Autodesk Inventor part; units mm, degrees
ref_plane "YZ Plane" through (0, 0, 0) normal (1, 0, 0) x (0, 1, 0)
ref_plane "XZ Plane" through (0, 0, 0) normal (0, 1, 0) x (-1, 0, 0)
ref_plane "XY Plane" through (0, 0, 0) normal (0, 0, 1) x (1, 0, 0)
sketch "Sketch1" plane through (0, 0, 0) normal (0, 0, 1) x (1, 0, 0)
  line L0 (0, 0) -> (40, 0)
  line L1 (40, 0) -> (40, 10)
  line L2 (40, 10) -> (0, 10)
  line L3 (0, 10) -> (0, 0)
  dimension "d0" = 40
  dimension "d1" = 10
extrude "Extrusion1" add sketch "Sketch1" along normal blind 10
sketch "Sketch2" plane through (0, 0, 10) normal (0, 0, 1) x (1, 0, 0)
  line L0 (0, 10) -> (0, 0)
  line L1 (40, 10) -> (0, 10)
  point P0 (5, 5)
  point P1 (35, 5)
  dimension "d4" = 30
  dimension "d5" = 5
  dimension "d6" = 5
  dimension "d7" = 5
hole "Hole1" at (5, 5, 10) at (35, 5, 10) direction (0, 0, -1) diameter 6 depth 5 tip angle 118
sketch "Sketch3" plane through (0, 0, 0) normal (0, 0, -1) x (-1, 0, 0)
  line L0 (0, 0) -> (-40, 0)
  line L1 (0, 10) -> (0, 0)
  line L2 (-40, 10) -> (0, 10)
  line L3 (-40, 0) -> (-40, 10)
extrude "Extrusion2" add sketch "Sketch3" along normal blind 10
sketch "Sketch4" plane through (0, 0, 10) normal (0, -1, 0) x (1, 0, 0)
  line L0 (40, -20) -> (0, -20)
  line L1 (0, -20) -> (0, -23)
  line L2 (0, -23) -> (40, -23)
  line L3 (40, -23) -> (40, -20)
  point P0 (0, -10)
  dimension "d17" = 3
extrude "Extrusion3" add sketch "Sketch4" against normal blind 52
sketch "Sketch5" plane through (40, 0, -13) normal (0, 0, -1) x (-1, 0, 0)
  line L0 (0, 52) -> (40, 52)
  line L1 (40, 52) -> (40, 62)
  line L2 (40, 62) -> (0, 62)
  line L3 (0, 62) -> (0, 52)
  point P0 (40, 0)
  dimension "d20" = 10
extrude "Extrusion4" add sketch "Sketch5" against normal up to surface (23 mm away)
sketch "Sketch6" plane through (0, 10, 10) normal (0, 1, 0) x (1, 0, 0)
  line L0 (0, 20) -> (0, 0)
  line L1 (40, 0) -> (0, 0)
  line L2 (40, 20) -> (40, 0)
  line L3 (0, 20) -> (40, 20)
  point P0 (0, 10)
extrude "Extrusion5" add sketch "Sketch6" along normal blind 22
sketch "Sketch7" plane through (0, 0, 10) normal (0, 0, 1) x (1, 0, 0)
  circle A0 centre (5, 5) radius 3
  circle A1 centre (35, 5) radius 3
  line L0 (0, 0) -> (40, 0)
  line L1 (40, 0) -> (40, 32)
  line L2 (0, 32) -> (40, 32)
  line L3 (0, 0) -> (0, 32)
  line L4 (0, 52) -> (0, 62)
  line L5 (40, 52) -> (0, 52)
  line L6 (40, 62) -> (40, 52)
  line L7 (0, 62) -> (40, 62)
extrude "Extrusion6" add sketch "Sketch7" along normal blind 10
properties part number "rail mount"
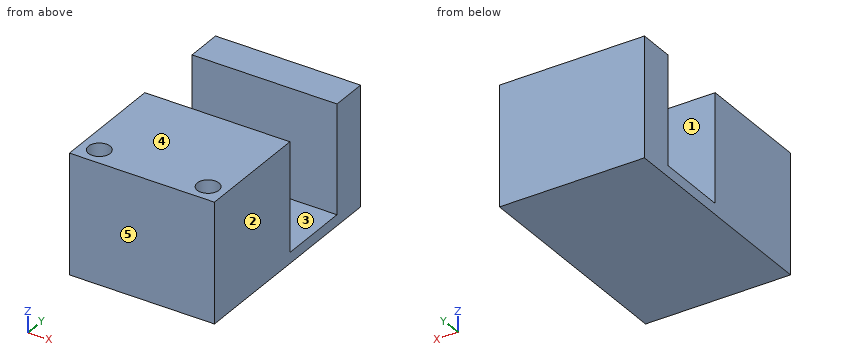
Design review of the part built by this model. Coordinates are the model's own, in mm. Face numbers are marked on the shaded views. A direction names the side the tool comes from. Round coordinates to 2 decimals unless told otherwise and drop trailing zeros. Write each loop counter-clockwise with the first axis right and the second up, starting at its lowest first coordinate (ties: lowest second). Pieces come first, ordered by that corner, then holes.
Item 1: Consider section D-D on y = 48.5. Give the boundary of the cut face in (x, z), and give its area (3 significant figures).
Item 2: For the marked faces 1 and 2, list the 3-axis set-ups (+Z, -Z, +X, -X, +Y, -Y) from which the entire face can be reached by the end or side of a thin tool; tool diameter is ignored.
Item 3: Consider section B-B on z = -4. Give the boundary of the cut face in (x, y).
Item 4: Consider section A-A on z = 15. Give the boundary of the cut face in (x, y), and give its area (3 significant figures).
Item 5: Wall thickness on L1, parallel to Y at x = 35, z = 8; L2, parallel to X at y = 5, z = 17; L3, parallel to Y at x = 28, z = 7.5: over which ranges is each line inside the solid? List them lowest first.
Item 6: For pin 1 Ø10 at (x, y) = (16, 46) entering from +Z, flat-tipped, find the tip position at first contact; note if it passes through.
Item 7: Consider section C-C on x = 16. Give the boundary of the cut face in (y, z), and give its area (3 significant figures).
Item 8: Draft analysis for pull direction Y (two halves, no side actions). For the marked faces 3, 4 and 5, state which applies: released by +Y, released by -Y, zero draft, split by the parting line, or undercut.
Check values:
1. outline: (0, -13) - (40, -13) - (40, -10) - (0, -10) - close
1. area: 120 mm2
2. face 1: +Z, +X, -X
2. face 2: +Z, -Z, +X, +Y, -Y
3. outline: (0, 0) - (40, 0) - (40, 32) - (0, 32) - close; (0, 52) - (40, 52) - (40, 62) - (0, 62) - close
4. outline: (0, 0) - (40, 0) - (40, 32) - (0, 32) - close; (0, 52) - (40, 52) - (40, 62) - (0, 62) - close; hole circle Ø6 at (5, 5); hole circle Ø6 at (35, 5)
4. area: 1,620 mm2
5. L1: y = 0 to 2, 8 to 32, 52 to 62
5. L2: x = 0 to 2, 8 to 32, 38 to 40
5. L3: y = 0 to 32, 52 to 62
6. pin 1: stops at z = -10
7. outline: (0, -13) - (62, -13) - (62, 20) - (52, 20) - (52, -10) - (32, -10) - (32, 20) - (0, 20) - close
7. area: 1,450 mm2
8. face 3: undercut
8. face 4: zero draft
8. face 5: released by -Y
